Source: CAD feature listing. Evaluate the final solid. Frame: model axes, mm. Face numbers are marked on the shaded views. A direction names the side the tool comes from. Round coordinates to 2 decimals unless told otherwise and drop trailing zeros. Order: outer loops, then holes, each group sorted by start corner. A loop starts at its lowest first (then second) coordinate and runs counter-clockwise, first axis right, second up. Notation, with made-up numbers: (-33.5, 37.5) -> (22.5, 37.5) arc R21 cw to (22.5, 41.5) -> close; hole circle Ø9 at (-3, -29). An arc over 180 degrees is marked (long way). Write item = value, one per line. Start each with the question number.
(1) Ray query, line 1 (Z direction, x = 35, y = -15.75); line 2 (Z direction, x = 44.5, y = -21) (3 decimals); line 3 (X direction, y = -2.5, z = 22.5). Return the intervals inside material, ascending.
(2) Draft query along Z for the marked faces 1, 2 and 3. Return one class per face: released by +Z, released by -Z, zero draft, split by the parting line, or undercut.
(3) Reachability of the marked faces 4 and 5 from +Z, -Z, +X, -X, +Y, -Y: full face, straight path, thin tool, end or side. Return the list, or none.
(4) Cut plane C-C on y = -17.75. Return the cut outline in (x, z).
(5) Contact query for flat-ended pins moving along their axis: pin 1 Ø2 at (x, y) = (-29.5, -14.5) entering from +Z; pin 2 Ø3 at (y, z) = (-15.5, 21.5) entering from -X; pin 3 Ø1 at (x, y) = (30.5, -8) entering from +Z. Output: stop coordinate, or through.
(6) Cut plane D-D on x = 36. Return the cut outline in (y, z).
(7) Cut plane B-B on z = 21. Return the cut outline in (x, y), then the cut area to 3 significant figures.
(8) Cut plane A-A on x = 3. Return the cut outline in (y, z), then the cut area to 3 significant figures.
from build123d import *

# Parameters (mm, degrees)
F0_R     = 30
F1_DEPTH = 25


with BuildPart() as f1:
    # F0 (on Front) → F1 (new body)
    with BuildSketch(Plane.XZ):
        with BuildLine():
            ThreePointArc((-9.8709988717, 44.4664797866), (-9.6765479631, 39.9795085396), (-11.9125396102, 36.0845035997))
            ThreePointArc((-11.9125396102, 36.0845035997), (-27.0421470159, 24.2777678435), (-37.1553505028, 7.9674292602))
            ThreePointArc((-37.1553505028, 7.9674292602), (-44.036048411, 1.0836405197), (-39.8366623459, -7.6967756324))
            ThreePointArc((-39.8366623459, -7.6967756324), (-35.6999774991, -15.297082174), (-42.3349477351, -20.8517190672))
            ThreePointArc((-42.3349477351, -20.8517190672), (-55.3349477351, -33.8517190672), (-42.3349477351, -46.8517190672))
            Line((-42.3349477351, -46.8517190672), (34.6360049196, -46.8517190672))
            ThreePointArc((34.6360049196, -46.8517190672), (47.5210264522, -35.5768915526), (38.0558333228, -21.3095990832))
            ThreePointArc((38.0558333228, -21.3095990832), (33.4543868939, -19.5118063183), (30.786217704, -15.3541337437))
            ThreePointArc((30.786217704, -15.3541337437), (24.3583291, -24.2942879499), (15.4351278274, -30.7456899823))
            ThreePointArc((15.4351278274, -30.7456899823), (16.8378076077, -32.4009903223), (17.3415790067, -34.5113798976))
            ThreePointArc((17.3415790067, -34.5113798976), (12.1247193284, -39.1518231188), (8.1239473631, -33.4296590287))
            ThreePointArc((8.1239473631, -33.4296590287), (-19.4089792265, -28.4047909501), (-34.0963191618, -4.5805723603))
            ThreePointArc((-34.0963191618, -4.5805723603), (-40.2756080675, -0.3812017982), (-34.1769117208, 3.9343778115))
            ThreePointArc((-34.1769117208, 3.9343778115), (-19.9809519782, 28.0053955797), (7.3990994056, 33.5975289496))
            ThreePointArc((7.3990994056, 33.5975289496), (10.830759038, 40.0793765069), (16.5063219502, 35.4340970516))
            ThreePointArc((16.5063219502, 35.4340970516), (15.8808188237, 33.0810127965), (14.1694376368, 31.3491253561))
            ThreePointArc((14.1694376368, 31.3491253561), (27.1897380489, 21.0774469129), (33.8915853443, 5.9077124496))
            ThreePointArc((33.8915853443, 5.9077124496), (38.9210173699, 6.9384879734), (41.7815475753, 2.6752671693))
            ThreePointArc((41.7815475753, 2.6752671693), (39.2225245159, -1.4515862058), (34.38826426, -0.9939339614))
            ThreePointArc((34.38826426, -0.9939339614), (34.1710361171, -3.985086476), (33.6941290984, -6.9459547822))
            ThreePointArc((33.6941290984, -6.9459547822), (35.7555321816, -5.8176755547), (38.0558333228, -5.3370391578))
            ThreePointArc((38.0558333228, -5.3370391578), (46.2747957775, 2.659963746), (38.0558333228, 10.6569666498))
            ThreePointArc((38.0558333228, 10.6569666498), (33.5332006387, 17.8616815332), (38.0558333228, 25.0663964165))
            ThreePointArc((38.0558333228, 25.0663964165), (48.5844980046, 36.975853683), (38.0558333228, 48.8853109494))
            Line((38.0558333228, 48.8853109494), (13.0399948809, 51.975853683))
            ThreePointArc((13.0399948809, 51.975853683), (1.5844980046, 63.4313505593), (-9.8709988717, 51.975853683))
            Line((-9.8709988717, 51.975853683), (-9.8709988717, 44.4664797866))
        make_face()
        with BuildLine():
            ThreePointArc((15.4351278274, -30.7456899823), (24.3583291, -24.2942879499), (30.786217704, -15.3541337437))
            ThreePointArc((30.786217704, -15.3541337437), (30.9635483069, -10.7085321739), (33.6941290984, -6.9459547822))
            ThreePointArc((33.6941290984, -6.9459547822), (34.1710361171, -3.985086476), (34.38826426, -0.9939339614))
            ThreePointArc((34.38826426, -0.9939339614), (32.5791661443, 2.3445688104), (33.8915853443, 5.9077124496))
            ThreePointArc((33.8915853443, 5.9077124496), (27.1897380489, 21.0774469129), (14.1694376368, 31.3491253561))
            ThreePointArc((14.1694376368, 31.3491253561), (10.2739993221, 30.9368169475), (7.3990994056, 33.5975289496))
            ThreePointArc((7.3990994056, 33.5975289496), (-19.9809519782, 28.0053955797), (-34.1769117208, 3.9343778115))
            ThreePointArc((-34.1769117208, 3.9343778115), (-32.0065217205, 2.2701500151), (-31.1837948135, -0.3381765267))
            ThreePointArc((-31.1837948135, -0.3381765267), (-31.9820022181, -2.9111475958), (-34.0963191618, -4.5805723603))
            ThreePointArc((-34.0963191618, -4.5805723603), (-19.4089792265, -28.4047909501), (8.1239473631, -33.4296590287))
            ThreePointArc((8.1239473631, -33.4296590287), (11.0591409817, -30.1253010368), (15.4351278274, -30.7456899823))
        make_face()
        Circle(F0_R, mode=Mode.SUBTRACT)
        with BuildLine():
            ThreePointArc((33.6941290984, -6.9459547822), (30.9635483069, -10.7085321739), (30.786217704, -15.3541337437))
            ThreePointArc((30.786217704, -15.3541337437), (32.5131227245, -11.2444419264), (33.6941290984, -6.9459547822))
        make_face()
    extrude(amount=F1_DEPTH)


solid = f1.part
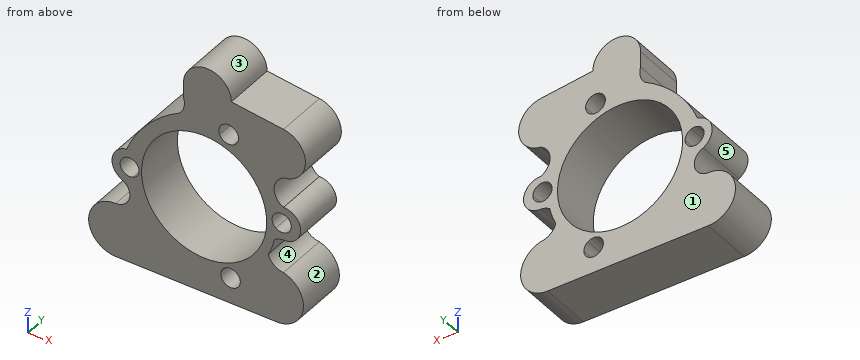
Evaluation:
q1.line_1 = -46.85 to -20.51, -6.14 to -1.39, 6.74 to 13.24, 22.48 to 49.26
q1.line_2 = -42.319 to -25.384, -2.365 to 7.685, 27.957 to 45.995
q1.line_3 = -28.57 to -19.84, 19.84 to 35.02
q2.face_1 = zero draft
q2.face_2 = undercut
q2.face_3 = released by +Z
q3.face_4 = +X, +Y, -Y
q3.face_5 = -X, +Y, -Y
q4.outline = (-42.33, -46.85) -> (34.64, -46.85) arc R13 ccw to (38.06, -21.31) arc R8 cw to (30.79, -15.35) arc R34.4 ccw to (33.69, -6.95) arc R8 cw to (38.06, -5.34) arc R8 ccw (long way) to (38.06, 10.66) arc R8 cw to (38.06, 25.07) arc R12 ccw to (38.06, 48.89) -> (13.04, 51.98) arc R11.46 ccw to (-9.87, 51.98) -> (-9.87, 44.47) arc R8.06 cw to (-11.91, 36.08) arc R54.63 ccw to (-37.16, 7.97) arc R8.43 ccw to (-39.84, -7.7) arc R6.83 cw to (-42.33, -20.85) arc R13 ccw to start; hole circle Ø9.09 at (-35.73, -0.34); hole circle Ø60 at (0, 0); hole circle Ø9.48 at (11.77, 35.43); hole circle Ø9.34 at (12.67, -34.51); hole circle Ø9.21 at (37.17, 2.68)
q5.pin_1 = 22.59
q5.pin_2 = -30.51
q5.pin_3 = 49.88
q6.outline = (-25, -46.78) -> (0, -46.78) -> (0, -20.91) -> (-25, -20.91) -> close; (-25, -5.73) -> (0, -5.73) -> (0, -1.78) -> (-25, -1.78) -> close; (-25, 7.13) -> (0, 7.13) -> (0, 12.08) -> (-25, 12.08) -> close; (-25, 23.64) -> (0, 23.64) -> (0, 49.14) -> (-25, 49.14) -> close
q7.outline = (-29.76, -25) -> (-21.42, -25) -> (-21.42, 0) -> (-29.76, 0) -> close; (21.42, -25) -> (34.17, -25) -> (34.17, 0) -> (21.42, 0) -> close
q7.area = 527 mm^2
q8.outline = (-25, -46.85) -> (0, -46.85) -> (0, -29.85) -> (-25, -29.85) -> close; (-25, 29.85) -> (0, 29.85) -> (0, 63.34) -> (-25, 63.34) -> close
q8.area = 1,260 mm^2
